Verification items for the finished model (mm, model axes). Face numbers are marked on the shaded views. A direction names the side the tool comes from. Give positions to 0.01 mm unless a question says otherwise; leave off trailing zeros. Loops run counter-clockwise (first coordinate to the right, second up) from the corner with the lowest first, then second, coordinate; pieces in that order, holes last. Notation, with made-up numbers: (50, 5) - (71, 5) arc R20 cw to (71, 27) - close; hole circle Ø4 at (-28.5, 53). An arc over 180 degrees is marked (long way). Answer in a Markdown table with one row per item.
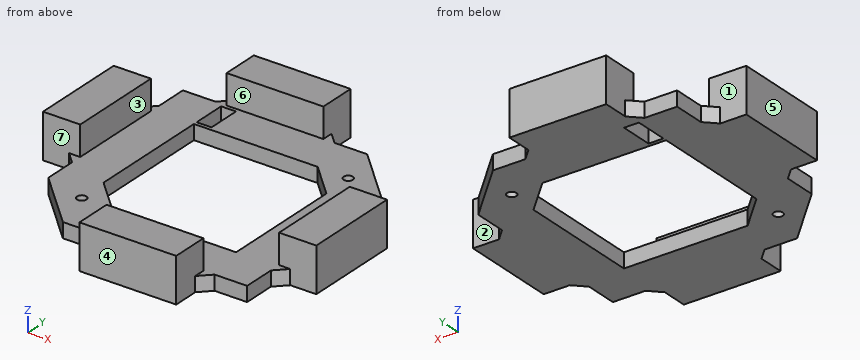
```python
from build123d import *

# Parameters (mm, degrees)
F1_DEPTH = 4
F2_R     = 1.25
F3_DEPTH = 4.001
F4_W     = 4
F4_H     = 9
F5_DEPTH = 4.001
F6_W     = 10
F6_H     = 26
F6_W_2   = 26
F6_H_2   = 10
F7_DEPTH = 12
F8_SIZE  = 3


with BuildPart() as f1:
    # F0 (on Top) → F1 (new body)
    with BuildSketch(Plane.XY):
        Polygon((17.4974746831, 32), (-32, 32), (-32, -17.4974746831), (-17.4974746831, -32), (32, -32), (32, 17.4974746831), align=None)
        Polygon((-21, -12.2340187158), (-21, 21), (12.2340187158, 21), (21, 21), (21, 12.2340187158), (21, -21), (-12.2340187158, -21), (-21, -21), align=None, mode=Mode.SUBTRACT)
        Polygon((-12.2340187158, -21), (-21, -12.2340187158), (-21, -21), align=None)
        Polygon((21, 21), (12.2340187158, 21), (21, 12.2340187158), align=None)
    extrude(amount=F1_DEPTH)

    # F2 (on face) → F3 (cut, through all)
    with BuildSketch(Plane.XY.offset(4)):
        with Locations((-20.6828733497, -20.6828733497)):
            Circle(F2_R)
        with Locations((20.6828733497, 20.6828733497)):
            Circle(F2_R)
    extrude(amount=-F3_DEPTH, mode=Mode.SUBTRACT)

    # F4 (on face) → F5 (cut, through all)
    with BuildSketch(Plane.XY.offset(4)):
        with Locations((-19, 26.5)):
            Rectangle(F4_W, F4_H)
    extrude(amount=-F5_DEPTH, mode=Mode.SUBTRACT)

    # F6 (on face) → F7 (join)
    with BuildSketch(Plane(origin=(0, 0, 0), x_dir=(1, 0, 0), z_dir=(0, 0, -1))):
        with Locations((-37, -7.2512626585)):
            Rectangle(F6_W, F6_H)
        with Locations((7.2512626585, 37)):
            Rectangle(F6_W_2, F6_H_2)
        with Locations((37, 7.2512626585)):
            Rectangle(F6_W, F6_H)
        with Locations((-7.2512626585, -37)):
            Rectangle(F6_W_2, F6_H_2)
    extrude(amount=-F7_DEPTH)

    # F8
    f8_edges = [f1.edges().sort_by_distance(p)[0] for p in [
        (32, 5.748737, 2),
        (32, -20.251263, 2),
        (20.251263, -32, 2),
        (-5.748737, -32, 2),
        (-32, -5.748737, 2),
        (-32, 20.251263, 2),
        (-20.251263, 32, 2),
        (5.748737, 32, 2),
    ]]
    chamfer(f8_edges, length=F8_SIZE)


solid = f1.part
```
Q1. Sectioned sample at A-A (x = -2). Record the cut outline in (y, z), and give its area (3 significant figures).
Completed:
| item | result |
|---|---|
| outline | (-42, 0) - (-21, 0) - (-21, 4) - (-32, 4) - (-32, 12) - (-42, 12) - close; (21, 0) - (42, 0) - (42, 12) - (32, 12) - (32, 4) - (21, 4) - close |
| area | 328 mm^2 |
Q2. Sectioned sample at D-D (x = 16). Record the cut outline in (y, z), and give its area (3 significant figures).
Completed:
| item | result |
|---|---|
| outline | (-42, 0) - (-21, 0) - (-21, 4) - (-32, 4) - (-32, 12) - (-42, 12) - close; (17.23, 0) - (32, 0) - (32, 4) - (17.23, 4) - close |
| area | 223 mm^2 |
Q3. Thickness scan on line 1 (X direction, y = -5.5, z = 9.25); line 2 (X direction, y = -20, z = 2). Record the ranges inside material, lowest first.
Completed:
| item | result |
|---|---|
| line 1 | -42 to -32, 32 to 42 |
| line 2 | -29.5 to -21.73, -19.64 to -13.23, 21 to 42 |
Q4. Go/stop test with flat-tipped pins: P1, Ø2, axis at x = -25.5, y = -15, coming from the +Z side; P2, Ø3, axis at y = -28, z = 2.5, coming from the +X side; P3, Ø10, axis at x = -5.5, y = 12, coming from the -Z side; P4, Ø3, axis at x = -20.68, y = -20.68, coming from the -Z side. Record where each tip stops, or that it passes through.
Completed:
| item | result |
|---|---|
| P1 | z = 4 |
| P2 | x = 32 |
| P3 | through |
| P4 | z = 0 |
Q5. Tool access check on the marked faces 1, 2, 3 and 4. Record the directions out of +Z, -Z, +X, -X, +Y, -Y that give a thin tool (end or side, any length) a straight path to the whole face; none if there is none.
Completed:
| item | result |
|---|---|
| face 1 | +Z, -X, +Y |
| face 2 | +Z, +X, +Y |
| face 3 | +Z, +Y, -Y |
| face 4 | +Z, -Z, +X, -X, -Y |
Q6. Sectioned sample at B-B (y = -11). Record the cut outline in (x, z).
Completed:
| item | result |
|---|---|
| outline | (-32, 0) - (-21, 0) - (-21, 4) - (-32, 4) - close; (21, 0) - (42, 0) - (42, 12) - (32, 12) - (32, 4) - (21, 4) - close |
Q7. Sectioned sample at C-C (z = 6.5). Record the cut outline in (x, y), and give its area (3 significant figures).
Completed:
| item | result |
|---|---|
| outline | (-42, -5.75) - (-32, -5.75) - (-32, 20.25) - (-42, 20.25) - close; (-20.25, 32) - (5.75, 32) - (5.75, 42) - (-20.25, 42) - close; (-5.75, -42) - (20.25, -42) - (20.25, -32) - (-5.75, -32) - close; (32, -20.25) - (42, -20.25) - (42, 5.75) - (32, 5.75) - close |
| area | 1,040 mm^2 |
Q8. Draft check along Y on the marked faces 5, 6 and 7. Enter one of: +Y half, -Y half, draft (parallel to the pull), parting line (faces both ways), or undercut.
Completed:
| item | result |
|---|---|
| face 5 | draft |
| face 6 | undercut |
| face 7 | -Y half |
